```python
from build123d import *

# Parameters (mm, degrees)
F1_DEPTH = 40
F2_R     = 2.5
F3_DEPTH = 25
F4_R     = 14
F5_DEPTH = 30
F6_R     = 7.5
F7_DEPTH = 20


with BuildPart() as f1:
    # F0 (on Top) → F1 (new body, symmetric)
    with BuildSketch(Plane.XY):
        with BuildLine():
            Line((-58, -104.5), (58, -104.5))
            ThreePointArc((58, -104.5), (61.5355339059, -103.0355339059), (63, -99.5))
            Line((63, -99.5), (63, 99.5))
            ThreePointArc((63, 99.5), (61.5355339059, 103.0355339059), (58, 104.5))
            Line((58, 104.5), (-58, 104.5))
            ThreePointArc((-58, 104.5), (-61.5355339059, 103.0355339059), (-63, 99.5))
            Line((-63, 99.5), (-63, -99.5))
            ThreePointArc((-63, -99.5), (-61.5355339059, -103.0355339059), (-58, -104.5))
        make_face()
    extrude(amount=F1_DEPTH, both=True)

    # F2 (on face) → F3 (cut)
    with BuildSketch(Plane(origin=(0, 0, -40), x_dir=(1, 0, 0), z_dir=(0, 0, -1))):
        with Locations((-53.5, -82)):
            Circle(F2_R)
        with Locations((53.5, -82)):
            Circle(F2_R)
        with Locations((-53.5, 68)):
            Circle(F2_R)
        with Locations((53.5, 68)):
            Circle(F2_R)
    extrude(amount=-F3_DEPTH, mode=Mode.SUBTRACT)

    # F4 (on face) → F5 (join)
    with BuildSketch(Plane.XZ.offset(104.5)):
        with Locations((-23, -5)):
            Circle(F4_R)
    extrude(amount=F5_DEPTH)

    # F6 (on face) → F7 (join)
    with BuildSketch(Plane(origin=(0, 104.5, 0), x_dir=(-1, 0, 0), z_dir=(0, 1, 0))):
        with Locations((-41.5932163596, 26.335991919)):
            Circle(F6_R)
        with Locations((43.447509408, 26.335991919)):
            Circle(F6_R)
    extrude(amount=F7_DEPTH)


solid = f1.part
```
Build history of the part. All positions in model axes, mm. A direction names the side the tool comes from. Round coordinates to 2 decimals unless told otherwise and drop trailing zeros. Write each loop counter-clockwise with the first axis right and the second up, starting at its lowest first coordinate (ties: lowest second). Pieces come first, ordered by that corner, then holes.
1) Band-saw the part on A-A, the plane x = -23. List the corners of the cut face in (y, z).
2) Mould opens along Y. For faces 5 (the cylindrical face through (-61.57, -103, 0.56)), 6 (the flat face through (42, 124.5, 26)), 7 (the flat face through (53, -68, -15)), 8 (the flat face through (-1, 1, 40)) say: +Y half, -Y half, draft (parallel to the pull), parting line (faces both ways), or undercut.
3) Drill centre lines: probe 1 along Y at (x, z) = (53.5, -30.5); probe 2 along X at (y, z) = (-68, -21.75); probe 3 along Y at (x, z) = (53, -34). Where is each one in solid material? Low to high.
4) 3-axis set-ups, long thin cutter, end or side, ignore diameter. For faces 1 (the cylindrical face through (-10.068, -119.29, -10.362)), 2 (the cylindrical face through (-37.92, 114.36, 31.405)), 3 (the flat face through (53, 82, -15)), 4 (the flat face through (-63, 1, 1)): which of +Z, -Z, +X, -X, +Y, -Y reach the whole face in a straight line?
5) Pin check, flat tips, straight feed: pin 1 (2 mm diameter, centred on x = 21, z = -24.5, fed in from +Y); pin 2 (2.5 mm diameter, centred on x = 54.5, y = 83, fed in from -Z); pin 3 (2 mm diameter, centred on x = -12.5, z = 25, fed in from -Y); pin 4 (2.5 mm diameter, centred on x = -54, y = 81.5, fed in from -Z). Stop position of each tip, or through.
6) Band-saw the part on D-D, the plane y = 82. List the corners of the cut face in (x, z), and give its area (3 significant figures).
7) Band-saw the part on C-C, the plane z = -5. List the corners of the cut face in (x, y), and give its area (3 significant figures).
8) Band-saw the part on B-B, the plane z = -21.5. List the corners of the cut face in (x, y).
Ans:
1. outline: (-134.5, -19) - (-104.5, -19) - (-104.5, -40) - (104.5, -40) - (104.5, 40) - (-104.5, 40) - (-104.5, 9) - (-134.5, 9) - close
2. face 5: -Y half
2. face 6: +Y half
2. face 7: undercut
2. face 8: draft
3. probe 1: y = -104.5 to -70.5, -65.5 to 79.5, 84.5 to 104.5
3. probe 2: x = -63 to -56, -51 to 51, 56 to 63
3. probe 3: y = -104.5 to -70.45, -65.55 to 79.55, 84.45 to 104.5
4. face 1: -Y
4. face 2: +Y
4. face 3: -Z
4. face 4: +Z, -Z, -X, +Y, -Y
5. pin 1: stops at y = 104.5
5. pin 2: stops at z = -40
5. pin 3: stops at y = -104.5
5. pin 4: stops at z = -15
6. outline: (-63, -40) - (-56, -40) - (-56, -15) - (-51, -15) - (-51, -40) - (51, -40) - (51, -15) - (56, -15) - (56, -40) - (63, -40) - (63, 40) - (-63, 40) - close
6. area: 9,830 mm2
7. outline: (-63, -99.5) arc R5 ccw to (-58, -104.5) - (-37, -104.5) - (-37, -134.5) - (-9, -134.5) - (-9, -104.5) - (58, -104.5) arc R5 ccw to (63, -99.5) - (63, 99.5) arc R5 ccw to (58, 104.5) - (-58, 104.5) arc R5 ccw to (-63, 99.5) - close
7. area: 27,200 mm2
8. outline: (-63, -99.5) arc R5 ccw to (-58, -104.5) - (58, -104.5) arc R5 ccw to (63, -99.5) - (63, 99.5) arc R5 ccw to (58, 104.5) - (-58, 104.5) arc R5 ccw to (-63, 99.5) - close; hole circle Ø5 at (-53.5, -68); hole circle Ø5 at (-53.5, 82); hole circle Ø5 at (53.5, -68); hole circle Ø5 at (53.5, 82)
